```python
from build123d import *

# Parameters (mm, degrees)
F0_R     = 6.35
F1_DEPTH = 25.4
F2_R     = 6.35
F3_DEPTH = 44.45
F4_SIZE  = 6.35


with BuildPart() as f1:
    # F0 (on Front) → F1 (new body)
    with BuildSketch(Plane.XZ):
        with BuildLine():
            Line((-22.402494, 12.7), (-86.464335, 12.7))
            Line((-86.464335, 12.7), (-86.464335, -12.7))
            Line((-86.464335, -12.7), (-22.964335, -12.7))
            ThreePointArc((-22.964335, -12.7), (-13.984079, -16.419744), (-10.264335, -25.4))
            ThreePointArc((-10.264335, -25.4), (-6.544591, -34.380256), (2.435665, -38.1))
            Line((2.435665, -38.1), (91.335665, -38.1))
            Line((91.335665, -38.1), (91.335665, -12.7))
            Line((91.335665, -12.7), (28.397506, -12.7))
            ThreePointArc((28.397506, -12.7), (19.41725, -8.980256), (15.697506, 0))
            ThreePointArc((15.697506, 0), (19.41725, 8.980256), (28.397506, 12.7))
            Line((28.397506, 12.7), (91.897506, 12.7))
            Line((91.897506, 12.7), (91.897506, 38.1))
            Line((91.897506, 38.1), (2.997506, 38.1))
            ThreePointArc((2.997506, 38.1), (-5.98275, 34.380256), (-9.702494, 25.4))
            ThreePointArc((-9.702494, 25.4), (-13.422238, 16.419744), (-22.402494, 12.7))
        make_face()
        with Locations((-73.764335, 0)):
            Circle(F0_R, mode=Mode.SUBTRACT)
    extrude(amount=F1_DEPTH)

    # F2 (on Top) → F3 (cut, symmetric)
    with BuildSketch(Plane.XY):
        with Locations((79.197506, -12.7)):
            Circle(F2_R)
    extrude(amount=F3_DEPTH, both=True, mode=Mode.SUBTRACT)

    # F4
    f4_edges = [f1.edges().sort_by_distance(p)[0] for p in [
        (91.897506, 0, 25.4),
        (91.335665, 0, -25.4),
        (91.897506, -25.4, 25.4),
        (91.335665, -25.4, -25.4),
    ]]
    chamfer(f4_edges, length=F4_SIZE)


solid = f1.part
```
Verification items for the finished model (mm, model axes). A direction names the side the tool comes from. Coordinates: 2 decimals unless noted, no trailing zeros. Loops run counter-clockwise (first coordinate to the right, second up) from the corner with the lowest first, then second, coordinate; pieces in that order, holes last. Notation, with made-up numbers: (14, -5.75) - (33, -5.75) arc R26 ccw to (33, 12.25) - close; hole circle Ø7 at (23, 9). An arc over 180 degrees is marked (long way). Put each result on its own line as item: value.
Item 1: Section check D-D (z = 31). Enter the section's corners in (x, y), then the cut area to 3 significant figures.
Conclusion:
outline: (-8.4, -25.4) - (85.55, -25.4) - (91.9, -19.05) - (91.9, -6.35) - (85.55, 0) - (-8.4, 0) - close; hole circle Ø12.7 at (79.2, -12.7)
area: 2,380 mm2
Item 2: Section check A-A (y = -12.7). Enter the section's corners in (x, z), then the cut area to 3 significant figures.
Conclusion:
outline: (-86.46, -12.7) - (-22.96, -12.7) arc R12.7 cw to (-10.26, -25.4) arc R12.7 ccw to (2.44, -38.1) - (72.85, -38.1) - (72.85, -12.7) - (28.4, -12.7) arc R12.7 cw to (28.4, 12.7) - (72.85, 12.7) - (72.85, 38.1) - (3, 38.1) arc R12.7 ccw to (-9.7, 25.4) arc R12.7 cw to (-22.4, 12.7) - (-86.46, 12.7) - close; (85.55, -38.1) - (91.34, -38.1) - (91.34, -12.7) - (85.55, -12.7) - close; (85.55, 12.7) - (91.9, 12.7) - (91.9, 38.1) - (85.55, 38.1) - close; hole circle Ø12.7 at (-73.76, 0)
area: 7,050 mm2
Item 3: Set-up check for faces 1 (the face through (-54, -13, 12.7)), 2 (the face through (88.205, -3.219, -25.578)), 3 (the face through (-55, -13, -12.7)): record each of +Z, -Z, +X, -X, +Y, -Y from which the full face is reachable in a straight line by a thin tool's end or side.
Conclusion:
face 1: +Z, -X, +Y, -Y
face 2: -Z, +X, +Y
face 3: -Z, -X, +Y, -Y
Item 4: Scan lines: line 1 along Z through (x, y) = (36.5, -12.75); line 2 along Z through (x, y) = (-29.5, -14); line 3 along Z through (x, y) = (-76, -13). Record each from-to range of solid material in increasing order.
Conclusion:
line 1: z = -38.1 to -12.7, 12.7 to 38.1
line 2: z = -12.7 to 12.7
line 3: z = -12.7 to -5.94, 5.94 to 12.7
Item 5: Section check B-B (z = 18). Enter the section's corners in (x, y), then the cut area to 3 significant figures.
Conclusion:
outline: (-12.08, -25.4) - (85.55, -25.4) - (91.9, -19.05) - (91.9, -6.35) - (85.55, 0) - (-12.08, 0) - close; hole circle Ø12.7 at (79.2, -12.7)
area: 2,470 mm2
Item 6: Section check C-C (x = -46.5). Enter the section's corners in (y, z).
Conclusion:
outline: (-25.4, -12.7) - (0, -12.7) - (0, 12.7) - (-25.4, 12.7) - close
Item 7: Draft check along Z on faces 4 (the face through (48, -13, 38.1)), 5 (the face through (60, -13, 12.7)), 6 (the face through (-86.464, -13, 0)), 7 (the face through (60, -13, -12.7)). Enter one of: pulls with the +Z half, pulls with the -Z half, needs draft (parallel to the pull), parting line crosses it, or undercut.
Conclusion:
face 4: pulls with the +Z half
face 5: undercut
face 6: needs draft
face 7: undercut
Item 8: Gauge pin test, flat ends, axial feed: pin 1 Ø10 at (x, y) = (79.2, -12.7) entering from +Z; pin 2 Ø2 at (x, z) = (19.5, 15) entering from +Y; pin 3 Ø4 at (x, y) = (-5.5, -16) entering from -Z; pin 4 Ø1 at (x, y) = (-29.5, -16) entering from +Z. Record the tip position at first contact, or that the pin passes through.
Conclusion:
pin 1: passes through
pin 2: stops at y = 0
pin 3: stops at z = -36.63
pin 4: stops at z = 12.7
